CAD build for the part. Positions are in the model's coordinates, mm. Round coordinates to 2 decimals unless told otherwise and drop trailing zeros. Loops run counter-clockwise (first coordinate to the right, second up) from the corner with the lowest first, then second, coordinate; pieces in that order, holes last. Notation, with made-up numbers: M 6,-6.75 L 63,-6.75 A30 cw 63,25.25 Z; hole C 27.5,34 d9. An arc over 180 degrees is marked long. Use a Markdown table: item, result. Add a question column.
(1) Wall check: L1, parallel to Z at x = 0, y = 3.5; L2, parallel to X at y = 58, z = 0.1; L3, parallel to Z at x = -0.6, y = 9. Give the ranges that are in metal, low to high.
(2) Flat gauge pin, fed straight in: P1, Ø2, axis at x = 0, z = 0, coming from the +Y side. Where does the tip first touch, or does it go through?
(3) Band-saw the part on B-B, the plane y = 48. Write the cut outline in (x, z), and give its area (3 significant figures).
(4) Band-saw the part on A-A, the plane y = 56. Write the cut outline in (x, z), and give its area (3 significant figures).
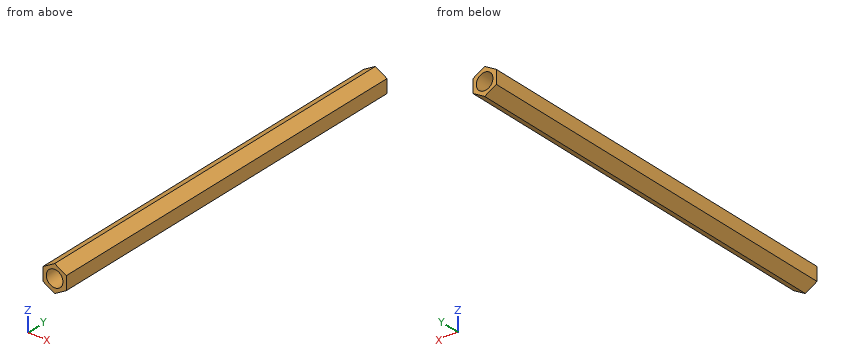
from build123d import *

# Parameters (mm, degrees)
BOSS_EXTRUDE1_DEPTH       = 60
M3X0_5_TAPPED_HOLE1_D     = 2.5
M3X0_5_TAPPED_HOLE1_DEPTH = 10
M3X0_5_TAPPED_HOLE1_TIP   = 0.751075774
M3X0_5_TAPPED_HOLE2_D     = 2.5
M3X0_5_TAPPED_HOLE2_DEPTH = 10
M3X0_5_TAPPED_HOLE2_TIP   = 0.751075774


with BuildPart() as part:
    # Sketch1 → Boss-Extrude1 (new body)
    with BuildSketch(Plane(origin=(0, 0, 0), x_dir=(1, 0, 0), z_dir=(0, 1, 0))):
        Polygon((0, 2.020725942), (-1.75, 1.010362971), (-1.75, -1.010362971), (0, -2.020725942), (1.75, -1.010362971), (1.75, 1.010362971), align=None)
    extrude(amount=BOSS_EXTRUDE1_DEPTH)

    # M3x0.5 Tapped Hole1
    with Locations(Plane(origin=(0, 60, 0), x_dir=(1, 0, 0), z_dir=(0, 1, 0))):
        with Locations((0, 0)):
            Hole(M3X0_5_TAPPED_HOLE1_D / 2, depth=M3X0_5_TAPPED_HOLE1_DEPTH)
            with Locations((0, 0, -(M3X0_5_TAPPED_HOLE1_DEPTH + M3X0_5_TAPPED_HOLE1_TIP / 2))):  # 118° drill point
                Cone(0, M3X0_5_TAPPED_HOLE1_D / 2, M3X0_5_TAPPED_HOLE1_TIP, mode=Mode.SUBTRACT)

    # M3x0.5 Tapped Hole2
    with Locations(Plane(origin=(0, 0, 0), x_dir=(-1, 0, 0), z_dir=(0, -1, 0))):
        with Locations((0, 0)):
            Hole(M3X0_5_TAPPED_HOLE2_D / 2, depth=M3X0_5_TAPPED_HOLE2_DEPTH)
            with Locations((0, 0, -(M3X0_5_TAPPED_HOLE2_DEPTH + M3X0_5_TAPPED_HOLE2_TIP / 2))):  # 118° drill point
                Cone(0, M3X0_5_TAPPED_HOLE2_D / 2, M3X0_5_TAPPED_HOLE2_TIP, mode=Mode.SUBTRACT)


solid = part.part
Return value:
| question | item | result |
|---|---|---|
| 1 | L1 | -2.02 to -1.25, 1.25 to 2.02 |
| 1 | L2 | -1.75 to -1.25, 1.25 to 1.75 |
| 1 | L3 | -1.67 to -1.1, 1.1 to 1.67 |
| 2 | P1 | y = 49.85 |
| 3 | outline | M -1.75,-1.01 L 0,-2.02 L 1.75,-1.01 L 1.75,1.01 L 0,2.02 L -1.75,1.01 Z |
| 3 | area | 10.6 mm^2 |
| 4 | outline | M -1.75,-1.01 L 0,-2.02 L 1.75,-1.01 L 1.75,1.01 L 0,2.02 L -1.75,1.01 Z; hole C 0,0 d2.5 |
| 4 | area | 5.70 mm^2 |
